from build123d import *

# Parameters (mm, degrees)
BOSS_EXTRUDE1_DEPTH                  = 31.75
CUT_EXTRUDE1_START                   = 31.75
SKETCH2_OUTSIDE_W                    = 27.938
SKETCH2_OUTSIDE_H                    = 28.954
SKETCH2_OUTSIDE_R                    = 6.35
CUT_EXTRUDE1_DEPTH                   = 7.9375
SKETCH5_OUTSIDE_W                    = 27.938
SKETCH5_OUTSIDE_H                    = 28.954
SKETCH5_OUTSIDE_R                    = 6.35
CUT_EXTRUDE5_DEPTH                   = 7.9375
F_10_32_TAPPED_HOLE1_D               = 4.0386
F_10_32_TAPPED_HOLE1_DEPTH           = 12.02944
F_10_32_TAPPED_HOLE1_TIP             = 1.213317848
F_10_32_TAPPED_HOLE1_ON_FACE_2_D     = 4.0386
F_10_32_TAPPED_HOLE1_ON_FACE_2_DEPTH = 12.02944
F_10_32_TAPPED_HOLE1_ON_FACE_2_TIP   = 1.213317848


with BuildPart() as part:
    # Sketch1 → Boss-Extrude1 (new, symmetric)
    with BuildSketch(Plane.XY):
        with BuildLine():
            ThreePointArc((0.93173274, 6.79441227), (0, 6.858), (-0.93173274, 6.79441227))
            Line((-0.93173274, 6.79441227), (-5.41826726, 4.204110358))
            ThreePointArc((-5.41826726, 4.204110358), (-5.939202219, 3.429), (-6.35, 2.590301913))
            Line((-6.35, 2.590301913), (-6.35, -2.590301913))
            ThreePointArc((-6.35, -2.590301913), (-5.939202219, -3.429), (-5.41826726, -4.204110358))
            Line((-5.41826726, -4.204110358), (-0.93173274, -6.79441227))
            ThreePointArc((-0.93173274, -6.79441227), (0, -6.858), (0.93173274, -6.79441227))
            Line((0.93173274, -6.79441227), (5.41826726, -4.204110358))
            ThreePointArc((5.41826726, -4.204110358), (5.939202219, -3.429), (6.35, -2.590301913))
            Line((6.35, -2.590301913), (6.35, 2.590301913))
            ThreePointArc((6.35, 2.590301913), (5.939202219, 3.429), (5.41826726, 4.204110358))
            Line((5.41826726, 4.204110358), (0.93173274, 6.79441227))
        make_face()
    extrude(amount=BOSS_EXTRUDE1_DEPTH, both=True)

    # Sketch2 outside → Cut-Extrude1 (cut)
    with BuildSketch(Plane.XY.offset(CUT_EXTRUDE1_START)):
        Rectangle(SKETCH2_OUTSIDE_W, SKETCH2_OUTSIDE_H)
        Circle(SKETCH2_OUTSIDE_R, mode=Mode.SUBTRACT)
    extrude(amount=-CUT_EXTRUDE1_DEPTH, mode=Mode.SUBTRACT)

    # Sketch5 outside → Cut-Extrude5 (cut)
    with BuildSketch(Plane(origin=(0, 0, -31.75), x_dir=(-1, 0, 0), z_dir=(0, 0, -1))):
        Rectangle(SKETCH5_OUTSIDE_W, SKETCH5_OUTSIDE_H)
        with Locations(Location((0, 0, 0), (0, 0, 180))):
            Circle(SKETCH5_OUTSIDE_R, mode=Mode.SUBTRACT)
    extrude(amount=-CUT_EXTRUDE5_DEPTH, mode=Mode.SUBTRACT)

    # #10-32 Tapped Hole1
    with Locations(Plane(origin=(0, 0, -31.75), x_dir=(-1, 0, 0), z_dir=(0, 0, -1))):
        with Locations((0, 0)):
            Hole(F_10_32_TAPPED_HOLE1_D / 2, depth=F_10_32_TAPPED_HOLE1_DEPTH)
            with Locations((0, 0, -(F_10_32_TAPPED_HOLE1_DEPTH + F_10_32_TAPPED_HOLE1_TIP / 2))):  # 118° drill point
                Cone(0, F_10_32_TAPPED_HOLE1_D / 2, F_10_32_TAPPED_HOLE1_TIP, mode=Mode.SUBTRACT)

    # #10-32 Tapped Hole1 on face 2
    with Locations(Plane.XY.offset(31.75)):
        with Locations((0, 0)):
            Hole(F_10_32_TAPPED_HOLE1_ON_FACE_2_D / 2, depth=F_10_32_TAPPED_HOLE1_ON_FACE_2_DEPTH)
            with Locations((0, 0, -(F_10_32_TAPPED_HOLE1_ON_FACE_2_DEPTH + F_10_32_TAPPED_HOLE1_ON_FACE_2_TIP / 2))):  # 118° drill point
                Cone(0, F_10_32_TAPPED_HOLE1_ON_FACE_2_D / 2, F_10_32_TAPPED_HOLE1_ON_FACE_2_TIP, mode=Mode.SUBTRACT)


solid = part.part
Work out the finished part from the listing and answer in its coordinate system (mm). A direction names the side the tool comes from. Give positions to 0.01 mm unless a question says otherwise; leave off trailing zeros. Loops run counter-clockwise (first coordinate to the right, second up) from the corner with the lowest first, then second, coordinate; pieces in that order, holes last. Notation, with made-up numbers: (44, 66) - (95, 66) arc R23 cw to (95, 79) - close; hole circle Ø11 at (49.25, 20). An arc over 180 degrees is marked (long way). Answer in a Markdown table with one row per item. Add a question column.
Q1. Determine the mould class of faces 6 (the cylindrical face through (2.93, 5.634, -27.837)), 7 (the flat face through (0, 6.5, -23.812)), 8 (the cylindrical face through (-1.926, 0.607, 25.651)) for opening direction X: released by +X, released by -X, zero draft, split by the parting line, or undercut.
Q2. Each of these flat-tipped pins is pushed along its axis until it touches: P1, Ø3, axis at x = -3, z = -10, coming from the -Y side; P2, Ø1.1, axis at x = 1.5, y = -6.5, coming from the +Z side; P3, Ø3, axis at x = 3.5, z = 8.5, coming from the -Y side; P4, Ø3, axis at x = 0, y = 0, coming from the -Z side. Where does it stop, or does it pass through?
Q3. Consider line 1 along X through (y, z) = (0, 25.25). Determine where the line is inside the solid, lowest interval first.
Q4. A tool of negligible diameter and unlimited length cuts with its end or side. For faces 1 (the flat face through (-5.7, 3.2, 23.812)), 2 (the flat face through (0, 6.5, 23.812)), 3 (the flat face through (5.7, 3.2, -23.812)), 4 (the flat face through (5.7, 3.2, 23.812)), 5 (the flat face through (-2, 2, -31.75)), from which of +Z, -Z, +X, -X, +Y, -Y can it reach the whole face along a straight path? Write none if from no direction.
Q5. The part is cut by section B-B (x = 4.75). Determine the outline of the cut face in (y, z), and give its area (3 significant figures).
Q6. The part is cut by section A-A (z = -16.5). Determine the outline of the cut face in (x, y), and give its area (3 significant figures).
Q7. The part is cut by section C-C (z = -25.5). Determine the outline of the cut face in (x, y), and give its area (3 significant figures).
Solution:
| question | item | result |
|---|---|---|
| 1 | face 6 | split by the parting line |
| 1 | face 7 | zero draft |
| 1 | face 8 | undercut |
| 2 | P1 | stops at y = -6.47 |
| 2 | P2 | stops at z = 31.75 |
| 2 | P3 | stops at y = -6.18 |
| 2 | P4 | stops at z = -19.41 |
| 3 | line 1 | x = -6.35 to -2.02, 2.02 to 6.35 |
| 4 | face 1 | +Z, -X, +Y |
| 4 | face 2 | +Z, +Y |
| 4 | face 3 | -Z, +X, +Y |
| 4 | face 4 | +Z, +X, +Y |
| 4 | face 5 | -Z, +X, -X, +Y, -Y |
| 5 | outline | (-4.59, -23.81) - (-4.21, -23.81) - (-4.21, -31.75) - (4.21, -31.75) - (4.21, -23.81) - (4.59, -23.81) - (4.59, 23.81) - (4.21, 23.81) - (4.21, 31.75) - (-4.21, 31.75) - (-4.21, 23.81) - (-4.59, 23.81) - close |
| 5 | area | 571 mm² |
| 6 | outline | (-6.35, -2.59) arc R6.86 ccw to (-5.42, -4.2) - (-0.93, -6.79) arc R6.86 ccw to (0.93, -6.79) - (5.42, -4.2) arc R6.86 ccw to (6.35, -2.59) - (6.35, 2.59) arc R6.86 ccw to (5.42, 4.2) - (0.93, 6.79) arc R6.86 ccw to (-0.93, 6.79) - (-5.42, 4.2) arc R6.86 ccw to (-6.35, 2.59) - close |
| 6 | area | 137 mm² |
| 7 | outline | circle Ø12.7 at (0, 0); hole circle Ø4.04 at (0, 0) |
| 7 | area | 114 mm² |
